Source: CAD feature listing. Evaluate the final solid. Frame: model axes, mm. Give positions to 0.01 mm unless a question says otherwise; leave off trailing zeros. Loops run counter-clockwise (first coordinate to the right, second up) from the corner with the lowest first, then second, coordinate; pieces in that order, holes last. Notation, with made-up numbers: (11, 47.25) - (19, 47.25) arc R18 cw to (19, 67.25) - close; hole circle Ø6 at (38.25, -3). An arc over 180 degrees is marked (long way). Write each question's results on one line, items separated by ' | '. Start each with the question number.
(1) Cut plane A-A on x = 9. Return the cut outline in (y, z), then the cut area to 3 significant figures.
(2) Material intervals for line 1 along Y through (x, z) = (32, -32.5); line 2 along X through (y, z) = (3.75, 39); line 3 along Z through (x, y) = (16, 4), sorted ascending. Write a range as [from, to].
(3) Cut plane B-B on z = 0. Return the cut outline in (x, y) (3 decimals).
(4) Contact query for flat-ended pins moving along their axis: pin 1 (2.5 mm diameter, centred on y = -5.5, z = -0.5, fed in from -X) (3 decimals); pin 2 (0.8 mm diameter, centred on x = 22, y = -4, fed in from +Z); pin 3 (12 mm diameter, centred on x = -47, z = 13, fed in from -Y). Output: stop coordinate, or through.
(5) Cut plane C-C on x = -56. Return the cut outline in (y, z).
(6) Cut plane D-D on z = -22. Return the cut outline in (x, y).
from build123d import *

# Parameters (mm, degrees)
SKETCH_1_W      = 130
SKETCH_1_H      = 130
EXTRUDE_1_DEPTH = 5
SKETCH_2_W      = 1
SKETCH_2_H      = 17.945111322
EXTRUDE_2_DEPTH = 8
SKETCH_3_R      = 2.5
EXTRUDE_3_DEPTH = 43
CHAMFER_1_SIZE  = 2


with BuildPart() as part:
    # 草图1 → 凸台-拉伸1 (new body)
    with BuildSketch(Plane(origin=(0, 0, 0), x_dir=(1, 0, 0), z_dir=(0, 1, 0))):
        with Locations((-0.501834335, 0.116589736)):
            Rectangle(SKETCH_1_W, SKETCH_1_H)
    extrude(amount=EXTRUDE_1_DEPTH)

    # 草图2 → 凸台-拉伸2 (add)
    with BuildSketch(Plane.XZ):
        with Locations((21.735, 0)):
            Rectangle(SKETCH_2_W, SKETCH_2_H)
        with Locations((-21.735, 0)):
            Rectangle(SKETCH_2_W, SKETCH_2_H)
    extrude(amount=EXTRUDE_2_DEPTH)

    # 草图3 → 凸台-拉伸3 (add)
    with BuildSketch(Plane.ZY.offset(22.235)):
        with Locations((0, -3.784370538)):
            Circle(SKETCH_3_R)
    extrude(amount=-EXTRUDE_3_DEPTH)

    # 倒角1
    chamfer_1_edges = [part.edges().sort_by_distance(p)[0] for p in [
        (64.498165665, 5, -0.116589736),
        (-0.501834335, 5, -65.116589736),
        (-65.501834335, 5, -0.116589736),
        (-0.501834335, 5, 64.883410264),
    ]]
    chamfer(chamfer_1_edges, length=CHAMFER_1_SIZE)


solid = part.part
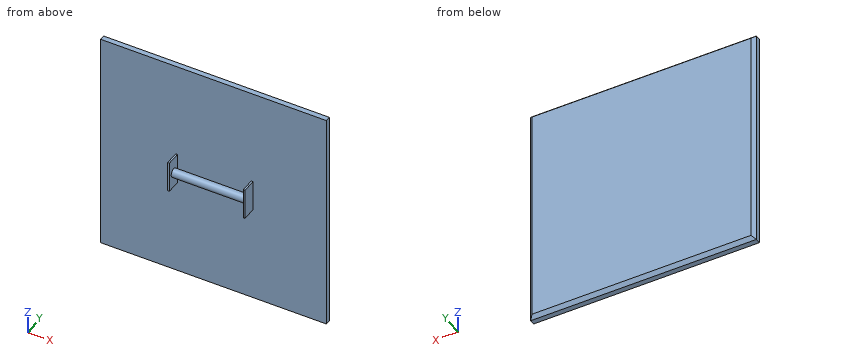
Ans:
1) outline: circle Ø5 at (-3.78, 0); (0, -65.12) - (3, -65.12) - (5, -63.12) - (5, 62.88) - (3, 64.88) - (0, 64.88) - close | area: 666 mm^2
2) line 1: [0, 5] | line 2: [-64.75, 63.75] | line 3: [-64.12, 63.88]
3) outline: (-65.502, 0) - (-22.235, 0) - (-22.235, -8) - (-21.235, -8) - (-21.235, -6.284) - (20.765, -6.284) - (20.765, -1.284) - (-21.235, -1.284) - (-21.235, 0) - (21.235, 0) - (21.235, -8) - (22.235, -8) - (22.235, 0) - (64.498, 0) - (64.498, 3) - (62.498, 5) - (-63.502, 5) - (-65.502, 3) - close
4) pin 1: x = -22.235 | pin 2: z = 8.97 | pin 3: y = 0
5) outline: (0, -65.12) - (3, -65.12) - (5, -63.12) - (5, 62.88) - (3, 64.88) - (0, 64.88) - close
6) outline: (-65.5, 0) - (64.5, 0) - (64.5, 3) - (62.5, 5) - (-63.5, 5) - (-65.5, 3) - close
